Geometry: final body of the model. Coordinates: model frame, mm. Face numbers are marked on the shaded views. Give positions to 0.01 mm unless a question says otherwise; leave off trailing zeros. Order: outer loops, then holes, each group sorted by start corner. A loop starts at its lowest first (then second) coordinate and runs counter-clockwise, first axis right, second up. Notation, with made-up numbers: (39, 56.5) - (90, 56.5) arc R9 ccw to (90, 68.5) - close; hole circle Ø5 at (1, -15). An arc over 180 degrees is marked (long way). Put each result on its own line as item: value. Start each with the question number.
1. First-contact query: P1, Ø2, axis at x = 6.5, z = 8.5, coming from the +Y side; P2, Ø2, axis at x = 11.5, z = 19, coming from the +Y side; P3, Ø4, axis at x = -5, z = 11, coming from the +Y side; P4, Ø12, axis at x = 12.5, y = -12.5, coming from the +Z side. Flat tips, straight axial feed; report the tip coordinate or a pass-through.
2. Mould query, pull axis Y, two halves, no side actions, for the marked faces 1, 2 and 3. Classes: pulls with the +Y half, pulls with the -Y half, needs draft (parallel to the pull), parting line crosses it, or undercut.
3. Section C-C on z = 13.5. Return the cut outline in (x, y), plus the area to 3 significant figures.
4. Ray query, line 1 along Y through (x, z) = (0, 9.25); line 2 along Y through (x, z) = (1.5, 11.75); line 3 along Z through (x, y) = (1, 9). Return the intervals inside material, ascending. Write a range as from..to.
5. Section A-A on x = 0. Return the cut outline in (y, z), plus the area to 3 significant figures.
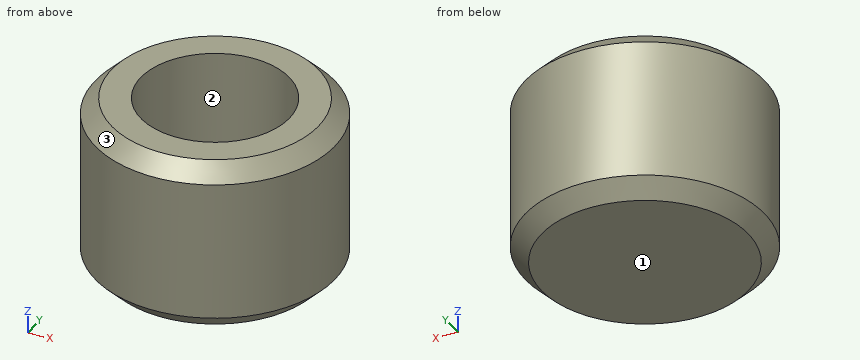
from build123d import *

# Parameters (mm, degrees)
F0_R     = 16.764
F0_R_2   = 10.414
F1_DEPTH = 22.86
F2_DEPTH = 1.27
F3_SIZE  = 2.286


with BuildPart() as f1:
    # F0 (on Top) → F1 (new body)
    with BuildSketch(Plane.XY):
        Circle(F0_R)
        Circle(F0_R_2, mode=Mode.SUBTRACT)
    extrude(amount=F1_DEPTH)

    # F0 (on Top) → F2 (join)
    with BuildSketch(Plane.XY):
        Circle(F0_R)
        Circle(F0_R_2, mode=Mode.SUBTRACT)
        Circle(F0_R_2)
    extrude(amount=-F2_DEPTH)

    # F3
    f3_edges = [f1.edges().sort_by_distance(p)[0] for p in [
        (-16.764, 0, -1.27),
        (-16.764, 0, 22.86),
    ]]
    chamfer(f3_edges, length=F3_SIZE)


solid = f1.part
Resolved:
1. P1: y = 15.84
1. P2: y = 13.07
1. P3: y = 16.49
1. P4: z = 22.86
2. face 1: needs draft
2. face 2: undercut
2. face 3: parting line crosses it
3. outline: circle Ø33.53 at (0, 0); hole circle Ø20.83 at (0, 0)
3. area: 542 mm^2
4. line 1: -16.76..-10.41, 10.41..16.76
4. line 2: -16.7..-10.31, 10.31..16.7
4. line 3: -1.27..0
5. outline: (-16.76, 1.02) - (-14.48, -1.27) - (14.48, -1.27) - (16.76, 1.02) - (16.76, 20.57) - (14.48, 22.86) - (10.41, 22.86) - (10.41, 0) - (-10.41, 0) - (-10.41, 22.86) - (-14.48, 22.86) - (-16.76, 20.57) - close
5. area: 322 mm^2
